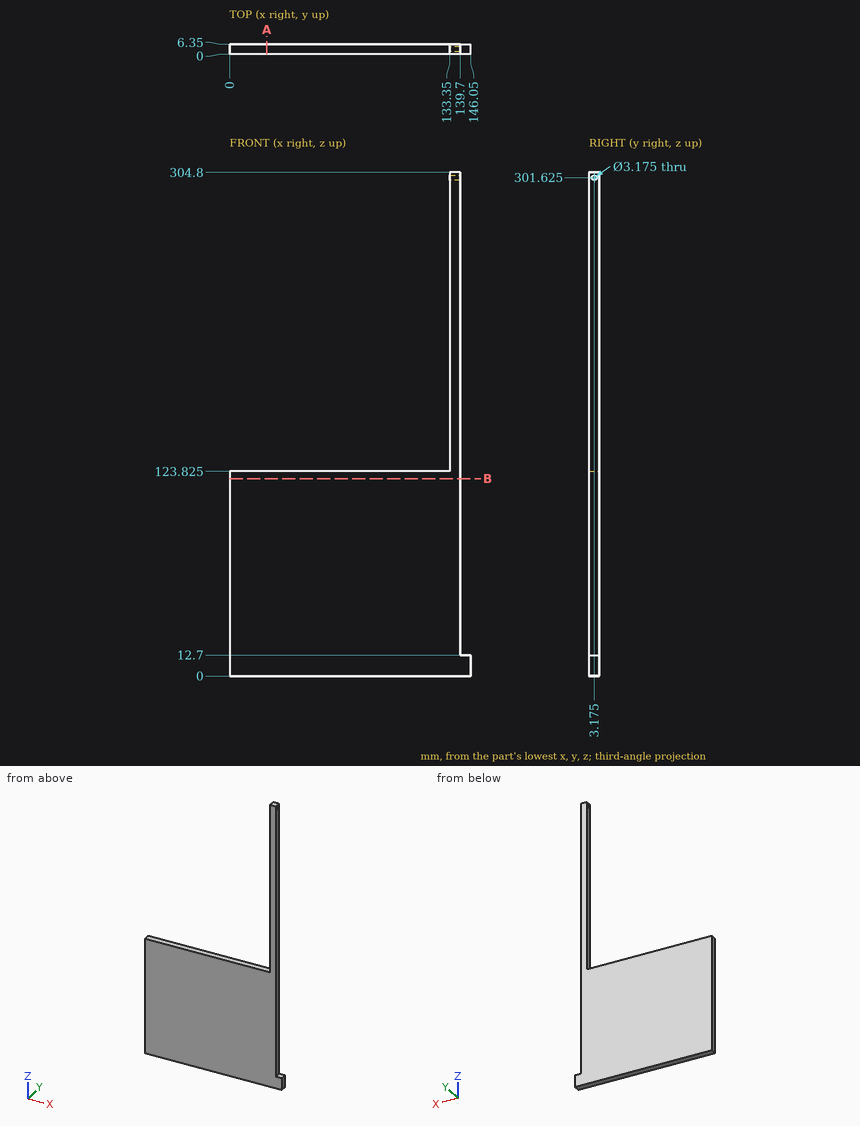
Design review of the part shown in the three views and the two pictorial views. Dimensions are in mm from the part's minimum x, y and z. Round coordinates to 2 decimals unless told otherwise and drop trailing zeros. Write each loop counter-clockwise with the first axis right and the second up, starting at its lowest first coordinate (ties: lowest second). Pieces come first, ordered by that corner, then holes. Notation, with made-up numbers: (0.5, -38.75) -> (14.5, -38.75) arc R35 cw to (14.5, -5.75) -> close; hole circle Ø3 at (65.5, -6.75). An arc over 180 degrees is marked (long way). Use one line per item in the form item = value.
1) Take a section at A-A, the plane x = 22.5. Write out the cut boundary in (y, z) (3 decimals).
Found:
outline = (0, 0) -> (6.35, 0) -> (6.35, 123.825) -> (0, 123.825) -> close
2) To check wall thickness, follow L1, parallel to X at y = 1.25, z = 134; L2, parallel to X at y = 3.5, z = 79; L3, parallel to Z at x = 67, y = 3.25 (3 decimals). State the ranges of each line that lie inside material, in increasing order. Write a range as from..to.
Found:
L1 = 133.35..139.7
L2 = 0..139.7
L3 = 0..123.825
3) Take a section at B-B, the plane z = 119.5. Write out the cut boundary in (x, y).
Found:
outline = (0, 0) -> (139.7, 0) -> (139.7, 6.35) -> (0, 6.35) -> close
4) Clearance check with flat-ended pins moving along their axes: pin 1 (2 mm diameter, centred on y = 1, z = 57.5, fed in from +X); pin 2 (3 mm diameter, centred on y = 3.175, z = 301.625, fed in from -X); pin 3 (1.9 mm diameter, centred on y = 2, z = 213.5, fed in from -X). State where each tip first meets the part, or that it passes through.
Found:
pin_1 = 139.7
pin_2 = through
pin_3 = 133.35
